from build123d import *

# Parameters (mm, degrees)
SKETCH3_R                 = 1.0795
CUT_EXTRUDE1_DEPTH        = 3.3749
CUT_EXTRUDE1_DEPTH_BACK   = 3.3749
SKETCH4_R                 = 1.0795
BOSS_EXTRUDE1_DEPTH       = 0.79375
SKETCH5_R                 = 2.3749
BOSS_EXTRUDE2_DEPTH       = 7.9375
F_4_40_TAPPED_HOLE1_D     = 2.2606
F_4_40_TAPPED_HOLE1_DEPTH = 12.7
F_4_40_TAPPED_HOLE1_TIP   = 0.679152758


with BuildPart() as part:
    # Sketch2 → Revolve1 (revolve)
    with BuildSketch(Plane.XY):
        with BuildLine():
            Line((0, 2.3749), (0, -2.3749))
            ThreePointArc((0, -2.3749), (2.3749, 0), (0, 2.3749))
        make_face()
    revolve(axis=Axis((0, 6.043929029, 0), (0, -1, 0)))

    # Sketch3 → Cut-Extrude1 (cut, two sides)
    with BuildSketch(Plane.XY) as cut_extrude1_sk:
        Circle(SKETCH3_R)
    extrude(amount=CUT_EXTRUDE1_DEPTH, mode=Mode.SUBTRACT)
    extrude(cut_extrude1_sk.sketch, amount=-CUT_EXTRUDE1_DEPTH_BACK, mode=Mode.SUBTRACT)

    # Sketch4 → Boss-Extrude1 (add, symmetric)
    with BuildSketch(Plane.XY):
        with BuildLine():
            Line((-3.175, 0), (-3.175, -4.7625))
            Line((-3.175, -4.7625), (-2.38125, -10.287))
            Line((-2.38125, -10.287), (2.38125, -10.287))
            Line((2.38125, -10.287), (3.175, -4.7625))
            Line((3.175, -4.7625), (3.175, 0))
            ThreePointArc((3.175, 0), (0, 3.175), (-3.175, 0))
        make_face()
        Circle(SKETCH4_R, mode=Mode.SUBTRACT)
    extrude(amount=BOSS_EXTRUDE1_DEPTH, both=True)

    # Sketch5 → Boss-Extrude2 (add, symmetric)
    with BuildSketch(Plane.XZ.offset(10.287)):
        Circle(SKETCH5_R)
    extrude(amount=BOSS_EXTRUDE2_DEPTH, both=True)

    # #4-40 Tapped Hole1
    with Locations(Plane(origin=(0, -18.2245, 0), x_dir=(-1, 0, 0), z_dir=(0, -1, 0))):
        with Locations((0, 0)):
            Hole(F_4_40_TAPPED_HOLE1_D / 2, depth=F_4_40_TAPPED_HOLE1_DEPTH)
            with Locations((0, 0, -(F_4_40_TAPPED_HOLE1_DEPTH + F_4_40_TAPPED_HOLE1_TIP / 2))):  # 118° drill point
                Cone(0, F_4_40_TAPPED_HOLE1_D / 2, F_4_40_TAPPED_HOLE1_TIP, mode=Mode.SUBTRACT)


solid = part.part
The listing builds one solid part. Answer for the finished solid, in the listing's coordinates (mm). A direction names the side the tool comes from. Round coordinates to 2 decimals unless told otherwise and drop trailing zeros. Write each loop counter-clockwise with the first axis right and the second up, starting at its lowest first coordinate (ties: lowest second). Pieces come first, ordered by that corner, then holes. Notation, with made-up numbers: M 35,71 L 84,71 A11 ccw 84,80 Z; hole C 11,54 d2. An arc over 180 degrees is marked long. Write each question's results on one line, items separated by ' | '. Start each with the question number.
(1) The part is cut by section C-C, the plane y = -8.25. Write down the section's boundary in (x, z).
(2) The part is cut by section B-B, the plane x = 2. Write down the section's boundary in (y, z).
(3) The part is cut by section A-A, the plane y = -6. Write down the section's boundary in (x, z).
(4) Determine the mould class of faces 4 (the flat face through (0, -2.35, -1)), 5 (the flat face through (-2.784, -7.486, 0.011)), 6 (the flat face through (-3.175, -2, 0)) for opening direction Y: +Y half, -Y half, draft (parallel to the pull), parting line (faces both ways), or undercut.
(5) Each of these flat-tipped pins is pushed along its axis until it touches: P1, Ø0.5, axis at x = 0, z = -1.5, coming from the +Y side; P2, Ø1.5, axis at x = 1.5, z = 2, coming from the +Y side; P3, Ø1, axis at y = -1, z = 2, coming from the +X side; P4, Ø1.3, axis at x = 0, y = 0, coming from the +Z side. Where does it stop, or does it pass through?
(6) Find the intervals of material crossed by line 1 (Y direction, x = 0, z = 0.9); line 2 (Z direction, x = 0, y = -8.25); line 3 (Y direction, x = 0.5, z = -1.75), in increasing order.
(7) For faces 1 (the flat face through (0, -2.35, 1)), 2 (the cylindrical face through (-0.51, -10.4, -2.32)), 3 (the cylindrical face through (1.03, 0.32, 0.03)), determine the directions among +Z, -Z, +X, -X, +Y, -Y from which every point of the face is accessible in a straight line to the end or side of a thin tool.
(8) The part is cut by section D-D, the plane y = -12. Write down the section's boundary in (x, z).
Worked answers:
1) outline: M -2.67,-0.79 L -2.24,-0.79 A2.37 ccw 2.24,-0.79 L 2.67,-0.79 L 2.67,0.79 L 2.24,0.79 A2.37 ccw -2.24,0.79 L -2.67,0.79 Z; hole C 0,0 d2.26
2) outline: M -18.22,-1.28 L -2.35,-1.28 L -2.35,-0.79 L -1.01,-0.79 A1.28 ccw 1.01,-0.79 L 2.47,-0.79 L 2.47,0.79 L 1.01,0.79 A1.28 ccw -1.01,0.79 L -2.35,0.79 L -2.35,1.28 L -18.22,1.28 Z
3) outline: M -3,-0.79 L -2.24,-0.79 A2.37 ccw 2.24,-0.79 L 3,-0.79 L 3,0.79 L 2.24,0.79 A2.37 ccw -2.24,0.79 L -3,0.79 Z; hole C 0,0 d2.26
4) face 4: undercut | face 5: -Y half | face 6: draft
5) P1: stops at y = 2.02 | P2: stops at y = 1.61 | P3: stops at x = 1.62 | P4: passes through
6) line 1: y = -5.39 to -2.35, -2.2 to -1.08, 1.08 to 2.2 | line 2: z = -2.37 to -1.13, 1.13 to 2.37 | line 3: y = -18.22 to -2.35, -1.53 to -0.96, 0.96 to 1.53
7) face 1: +Z, +X, -X | face 2: -Y | face 3: +Z, -Z
8) outline: C 0,0 d4.75; hole C 0,0 d2.26
